Autodesk Inventor part; units mm, degrees
ref_plane "YZ Plane" through (0, 0, 0) normal (1, 0, 0) x (0, 1, 0)
ref_plane "XZ Plane" through (0, 0, 0) normal (0, 1, 0) x (-1, 0, 0)
ref_plane "XY Plane" through (0, 0, 0) normal (0, 0, 1) x (1, 0, 0)
sketch "Sketch2" plane through (0, 0, 0) normal (0, 0, 1) x (1, 0, 0)
  line L0 (-25.4, -12.7) -> (25.4, -12.7)
  line L1 (25.4, -12.7) -> (25.4, 12.7)
  line L2 (25.4, 12.7) -> (-25.4, 12.7)
  line L3 (-25.4, 12.7) -> (-25.4, -12.7)
  line L4 (-25.4, -12.7) -> (25.4, 12.7) construction
  line L5 (25.4, -12.7) -> (-25.4, 12.7) construction
  point P0 (0, 0)
  dimension "d4" = 50.8
  dimension "d5" = 25.4
extrude "Extrusion2" add sketch "Sketch2" along normal mid plane 25.4
sketch "Sketch3" plane through (-25.4, 12.7, 12.7) normal (0, 1, 0) x (1, 0, 0)
  line L0 (0, 25.4) -> (0, 0) construction
  line L1 (25.4, 12.7) -> (25.4, 19.05)
  line L2 (25.4, 19.05) -> (0, 19.05)
  line L3 (0, 19.05) -> (0, 12.7)
  line L4 (0, 0) -> (0, 25.4) construction
  line L5 (25.4, 12.7) -> (25.4, 6.35)
  line L6 (25.4, 6.35) -> (0, 6.35)
  line L7 (0, 6.35) -> (0, 12.7)
  dimension "d8" = 25.4
  dimension "d10" = 12.7
extrude "Extrusion3" cut sketch "Sketch3" against normal through all
sketch "Sketch4" plane through (0, 0, 12.7) normal (0, 0, 1) x (1, 0, 0)
  circle A0 centre (-12.7, 0) radius 5.2705
  line L0 (-25.4, 12.7) -> (-25.4, -12.7)
  point P0 (0, 0)
  dimension "d13" = 10.541
  dimension "d14" = 12.7
extrude "Extrusion4" cut sketch "Sketch4" against normal through all
sketch "Sketch5" plane through (25.4, -12.7, 12.7) normal (1, 0, 0) x (0, 0, -1)
  circle A0 centre (12.7, 12.7) radius 4.2164
  dimension "d27" = 8.4328
extrude "Extrusion5" cut sketch "Sketch5" against normal blind 12.7
properties part number "piston" material "PET Plastic"
The model under review builds one solid part; all positions refer to its coordinate system, in mm. A direction names the side the tool comes from. Round coordinates to 2 decimals unless told otherwise and drop trailing zeros. Order: outer loops, then holes, each group sorted by start corner. A loop starts at its lowest first (then second) coordinate and runs counter-clockwise, first axis right, second up. Notation, with made-up numbers: (59, 59) -> (83, 59) arc R17 cw to (83, 75) -> close; hole circle Ø2 at (76.5, 9). An arc over 180 degrees is marked (long way). Use a Markdown table: item, result.
Q1. Tool access review of faces 5 (the flat face through (0, 0, 0)), 6 (the flat face through (-25.4, 0, 9)), 7 (the flat face through (12.7, 0, 0)): name each direction out of +Z, -Z, +X, -X, +Y, -Y from which nothing blocks a thin tool from reaching the whole face with its end or side.
Values:
| item | result |
|---|---|
| face 5 | -X, +Y, -Y |
| face 6 | +Z, -Z, -X, +Y, -Y |
| face 7 | +X |
Q2. We need section C-C on z = 8.25. Write out the cut boundary in (x, y).
Values:
| item | result |
|---|---|
| outline | (-25.4, -12.7) -> (25.4, -12.7) -> (25.4, 12.7) -> (-25.4, 12.7) -> close; hole circle Ø10.54 at (-12.7, 0) |
Q3. We need section D-D on x = 19. Write out the cut boundary in (y, z), then the cut area to 3 significant figures.
Values:
| item | result |
|---|---|
| outline | (-12.7, -12.7) -> (12.7, -12.7) -> (12.7, 12.7) -> (-12.7, 12.7) -> close; hole circle Ø8.43 at (0, 0) |
| area | 589 mm^2 |
Q4. Clearance check with flat-ended pins moving along their axes: P1, Ø9.5, axis at y = -2, z = 1, coming from the +X side; P2, Ø7.5, axis at y = 0, z = 0, coming from the -X side; P3, Ø9.5, axis at x = -12.7, y = 0, coming from the +Z side. State where each tip first meets the part, or that it passes through.
Values:
| item | result |
|---|---|
| P1 | stops at x = 25.4 |
| P2 | stops at x = 0 |
| P3 | passes through |
Q5. We need section B-B on y = 0. Write out the cut boundary in (x, z).
Values:
| item | result |
|---|---|
| outline | (-25.4, -12.7) -> (-17.97, -12.7) -> (-17.97, -6.35) -> (-25.4, -6.35) -> close; (-25.4, 6.35) -> (-17.97, 6.35) -> (-17.97, 12.7) -> (-25.4, 12.7) -> close; (-7.43, -12.7) -> (25.4, -12.7) -> (25.4, -4.22) -> (12.7, -4.22) -> (12.7, 4.22) -> (25.4, 4.22) -> (25.4, 12.7) -> (-7.43, 12.7) -> (-7.43, 6.35) -> (0, 6.35) -> (0, -6.35) -> (-7.43, -6.35) -> close |
Q6. Mouldability with a two-part tool opening along Z and no side actions: class faces 1 (the cylindrical face through (19.14, 4.18, 0.55)), 2 (the flat face through (0, 0, 12.7)), 3 (the flat face through (6, 12.7, 0)), 4 (the flat face through (0, 0, -12.7)) as +Z half, -Z half, draft (parallel to the pull), parting line (faces both ways), or undercut.
Values:
| item | result |
|---|---|
| face 1 | undercut |
| face 2 | +Z half |
| face 3 | draft |
| face 4 | -Z half |
Q7. We need section A-A on x = -22. Write out the cut boundary in (y, z).
Values:
| item | result |
|---|---|
| outline | (-12.7, -12.7) -> (12.7, -12.7) -> (12.7, -6.35) -> (-12.7, -6.35) -> close; (-12.7, 6.35) -> (12.7, 6.35) -> (12.7, 12.7) -> (-12.7, 12.7) -> close |
Q8. For line 1 (Z direction, x = -21, y = 1.5); line 2 (Y direction, x = -12.7, z = 11.25); line 3 (Z direction, x = 20, y = -0.75), list the stretches that pass through material, from the lowest coordinate up.
Values:
| item | result |
|---|---|
| line 1 | z = -12.7 to -6.35, 6.35 to 12.7 |
| line 2 | y = -12.7 to -5.27, 5.27 to 12.7 |
| line 3 | z = -12.7 to -4.15, 4.15 to 12.7 |
